Part model, mm, in its own coordinate system. Face numbers are marked on the shaded views. A direction names the side the tool comes from. Coordinates: 2 decimals unless noted, no trailing zeros. Order: outer loops, then holes, each group sorted by start corner. A loop starts at its lowest first (then second) coordinate and runs counter-clockwise, first axis right, second up.
1) Cut at C-C (z = -9). List the corners of the cut face in (x, y), and give its area (3 significant figures).
2) Wall check: L1, parallel to Z at x = 4, y = 45.5; L2, parallel to Y at x = 0, z = 21.75. Give the ranges that are in metal, low to high.
3) Cut at D-D (z = 16.5). List the corners of the cut face in (x, y).
4) Cut at A-A (x = 0). List the corners of the cut face in (y, z).
5) Tool access for the marked faces 4, 5 and 6: list every direction of +Z, -Z, +X, -X, +Y, -Y with a clear straight run to the whole face (end or side of a thin tool).
6) Cut at B-B (y = 31). List the corners of the cut face in (x, z), and give its area (3 significant figures).
7) Pin check, flat tips, straight feed: pin 1 Ø25 at (y, z) = (21.5, -11) entering from +X; pin 2 Ø0.8 at (x, z) = (22, -2) entering from +Y; pin 3 Ø3 at (x, z) = (-4, 0) entering from +Y. Stop position of each tip, or through.
8) Mould opens along X. For the marked faces 1, 2 and 3 say: +X half, -X half, draft (parallel to the pull), parting line (faces both ways), or undercut.
```python
from build123d import *

# Parameters (mm, degrees)
SKETCH1_W               = 50
SKETCH1_H               = 50
BOSS_EXTRUDE1_DEPTH     = 100
SKETCH4_R               = 2.5
BOSS_EXTRUDE2_DEPTH     = 4.5
CUT_EXTRUDE1_DEPTH      = 161.078105936
CUT_EXTRUDE1_DEPTH_BACK = 161.078105936
SKETCH5_R               = 2.5
SKETCH6_W               = 50
SKETCH6_H               = 50
CUT_EXTRUDE2_DEPTH      = 4.5
CHAMFER1_SIZE           = 2
CHAMFER2_SIZE           = 5
SKETCH7_W               = 41
SKETCH7_H               = 41
CUT_EXTRUDE3_DEPTH      = 45
SKETCH8_W               = 34
SKETCH8_H               = 41
CUT_EXTRUDE4_DEPTH      = 30
CUT_EXTRUDE5_DEPTH      = 34
SKETCH10_W              = 5
SKETCH10_H              = 50.266184812
CUT_EXTRUDE6_DEPTH      = 25


with BuildPart() as part:
    # Sketch1 → Boss-Extrude1 (new body)
    with BuildSketch(Plane(origin=(0, 0, 0), x_dir=(1, 0, 0), z_dir=(0, 1, 0))):
        Rectangle(SKETCH1_W, SKETCH1_H)
    extrude(amount=BOSS_EXTRUDE1_DEPTH)

    # Sketch4 → Boss-Extrude2 (add)
    with BuildSketch(Plane(origin=(0, 0, -25), x_dir=(-1, 0, 0), z_dir=(0, 0, -1))):
        with BuildLine():
            Line((-25, 100), (25, 100))
            Line((25, 100), (25, 125))
            ThreePointArc((25, 125), (0, 150), (-25, 125))
            Line((-25, 125), (-25, 100))
        make_face()
        with Locations((0, 125)):
            Circle(SKETCH4_R, mode=Mode.SUBTRACT)
    boss_extrude2 = extrude(amount=-BOSS_EXTRUDE2_DEPTH)

    # Mirror2: Boss-Extrude2 across plane
    add(boss_extrude2.mirror(Plane.XY))

    # Sketch5 → Cut-Extrude1 (cut, two sides: drawn at the far end of the back side and taken through both)
    with BuildSketch(Plane.ZY.offset(-25).offset(-CUT_EXTRUDE1_DEPTH_BACK)):
        with BuildLine():
            Line((-25, 0), (2.6e-08, 0))
            ThreePointArc((2.6e-08, 0), (-17.67766952, 7.322330461), (-25, 25))
            Line((-25, 25), (-25, 0))
        make_face()
        with BuildLine():
            Line((25, 0), (25, 25))
            ThreePointArc((25, 25), (17.677669539, 7.32233048), (2.6e-08, 0))
            Line((2.6e-08, 0), (25, 0))
        make_face()
        with Locations((0, 25)):
            Circle(SKETCH5_R)
    extrude(amount=CUT_EXTRUDE1_DEPTH + CUT_EXTRUDE1_DEPTH_BACK, mode=Mode.SUBTRACT)

    # Sketch6 → Cut-Extrude2 (cut)
    with BuildSketch(Plane(origin=(25, 0, 0), x_dir=(0, 0, -1), z_dir=(1, 0, 0))):
        with Locations((0, 25)):
            Rectangle(SKETCH6_W, SKETCH6_H)
    cut_extrude2 = extrude(amount=-CUT_EXTRUDE2_DEPTH, mode=Mode.SUBTRACT)

    # Mirror3: Cut-Extrude2 across plane
    add(cut_extrude2.mirror(Plane(origin=(0, 0, 0), x_dir=(0, 0, 1), z_dir=(1, 0, 0))), mode=Mode.SUBTRACT)

    # Chamfer1
    chamfer1_edges = [part.edges().sort_by_distance(p)[0] for p in [
        (-25, 100, 0),
        (0, 150, -25),
        (25, 100, 0),
        (0, 150, 25),
        (25, 87.5, 25),
        (-25, 87.5, 25),
        (-25, 87.5, -25),
        (25, 87.5, -25),
    ]]
    chamfer(chamfer1_edges, length=CHAMFER1_SIZE)

    # Chamfer2
    # the kernel refuses this chamfer: 5 mm, written as the material it takes off along each edge
    with BuildSketch(Plane(origin=(25, 50, 35.85841494), x_dir=(0.027495876610586317, 0.9996219169112968, 0), z_dir=(0, 0, -1))) as chamfer2_piece_1_section:
        Polygon((CHAMFER2_SIZE * 0.999621916911, -CHAMFER2_SIZE * 0.0274958766106), (-CHAMFER2_SIZE * 0.0274958766106, -CHAMFER2_SIZE * 0.999621916911), (0, 0), align=None)
    chamfer2_piece_1 = extrude(amount=71.71682988, mode=Mode.PRIVATE)
    chamfer2_piece_1 = split(chamfer2_piece_1, bisect_by=Plane(origin=(20.5, 51.679503735, 0), z_dir=(1, 0, 0)), keep=Keep.TOP, mode=Mode.PRIVATE)
    add(chamfer2_piece_1, mode=Mode.SUBTRACT)
    with BuildSketch(Plane(origin=(-25, 50, 35.85841494), x_dir=(-0.027495876610586317, 0.9996219169112968, 0), z_dir=(0, 0, -1))) as chamfer2_piece_2_section:
        Polygon((CHAMFER2_SIZE * 0.999621916911, CHAMFER2_SIZE * 0.0274958766106), (-CHAMFER2_SIZE * 0.0274958766106, CHAMFER2_SIZE * 0.999621916911), (0, 0), align=None)
    chamfer2_piece_2 = extrude(amount=71.71682988, mode=Mode.PRIVATE)
    chamfer2_piece_2 = split(chamfer2_piece_2, bisect_by=Plane(origin=(-20.5, 51.679503735, 0), z_dir=(-1, 0, 0)), keep=Keep.TOP, mode=Mode.PRIVATE)
    add(chamfer2_piece_2, mode=Mode.SUBTRACT)

    # Sketch7 → Cut-Extrude3 (cut)
    with BuildSketch(Plane(origin=(0, 100, 0), x_dir=(1, 0, 0), z_dir=(0, 1, 0))):
        Rectangle(SKETCH7_W, SKETCH7_H)
    extrude(amount=-CUT_EXTRUDE3_DEPTH, mode=Mode.SUBTRACT)

    # Sketch8 → Cut-Extrude4 (cut)
    with BuildSketch(Plane(origin=(0, 55, 0), x_dir=(1, 0, 0), z_dir=(0, 1, 0))):
        Rectangle(SKETCH8_W, SKETCH8_H)
    extrude(amount=-CUT_EXTRUDE4_DEPTH, mode=Mode.SUBTRACT)

    # Sketch9 → Cut-Extrude5 (cut)
    with BuildSketch(Plane.ZY.offset(-17)):
        with BuildLine():
            Line((-21, 25), (21, 25))
            ThreePointArc((21, 25), (0, 4), (-21, 25))
        make_face()
    extrude(amount=CUT_EXTRUDE5_DEPTH, mode=Mode.SUBTRACT)

    # Sketch10 → Cut-Extrude6 (cut)
    with BuildSketch(Plane(origin=(0, 0, 0), x_dir=(1, 0, 0), z_dir=(0, 1, 0))):
        Rectangle(SKETCH10_W, SKETCH10_H)
    extrude(amount=CUT_EXTRUDE6_DEPTH, mode=Mode.SUBTRACT)


solid = part.part
```
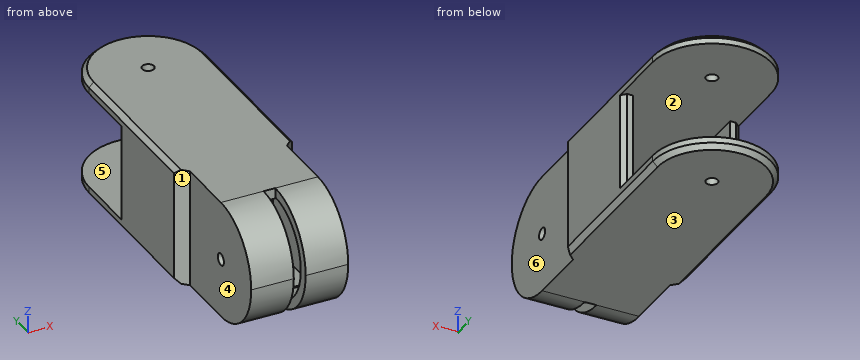
Geometry check:
1. outline: (-25, 55) - (-20.5, 50.5) - (-20.5, 1.68) - (-2.5, 1.68) - (-2.5, 6.03) - (-17, 6.03) - (-17, 55) - (-20.5, 55) - (-20.5, 100) - (-23, 100) - (-25, 98) - close; (2.5, 1.68) - (20.5, 1.68) - (20.5, 50.5) - (25, 55) - (25, 98) - (23, 100) - (20.5, 100) - (20.5, 55) - (17, 55) - (17, 6.03) - (2.5, 6.03) - close
1. area: 921 mm2
2. L1: z = -25 to -20.5, 20.5 to 25
2. L2: y = 25 to 122.5, 127.5 to 150
3. outline: (-25, 55) - (-20.5, 50.5) - (-20.5, 6.22) - (-2.5, 6.22) - (-2.5, 12.01) - (-17, 12.01) - (-17, 55) - (-20.5, 55) - (-20.5, 100) - (-23, 100) - (-25, 98) - close; (2.5, 6.22) - (20.5, 6.22) - (20.5, 50.5) - (25, 55) - (25, 98) - (23, 100) - (20.5, 100) - (20.5, 55) - (17, 55) - (17, 12.01) - (2.5, 12.01) - close
4. outline: (25, -25) - (122.5, -25) - (122.5, -20.5) - (25, -20.5) - close; (25, 20.5) - (122.5, 20.5) - (122.5, 25) - (25, 25) - close; (127.5, -25) - (148, -25) - (150, -23) - (150, -20.5) - (127.5, -20.5) - close; (127.5, 20.5) - (150, 20.5) - (150, 23) - (148, 25) - (127.5, 25) - close
5. face 4: +Z, -Z, -X, -Y
5. face 5: +Y
5. face 6: +Z, -Z, +X, -Y
6. outline: (-20.5, -25) - (20.5, -25) - (20.5, 25) - (-20.5, 25) - close; hole (-17, -20.5) - (17, -20.5) - (17, 20.5) - (-17, 20.5) - close
6. area: 656 mm2
7. pin 1: stops at x = 20.5
7. pin 2: stops at y = 100
7. pin 3: stops at y = 4.05
8. face 1: -X half
8. face 2: undercut
8. face 3: draft
